Verification items for the finished model (mm, model axes). Face numbers are marked on the shaded views. A direction names the side the tool comes from. Round coordinates to 2 decimals unless told otherwise and drop trailing zeros. Write each loop counter-clockwise with the first axis right and the second up, starting at its lowest first coordinate (ties: lowest second). Pieces come first, ordered by that corner, then holes. Notation, with made-up numbers: M 76.5,14 L 118.5,14 A20 ccw 118.5,28 Z; hole C 8.25,30 d5. An arc over 180 degrees is marked long. Answer in a Markdown table with one row per item. Add a question column.
1. Set-up check for the marked faces 1, 2 and 3: record each of +Z, -Z, +X, -X, +Y, -Y from which the full face is reachable in a straight line by a thin tool's end or side.
2. Material ranges on probe 1 along Y at (x, z) = (38.5, 1.35); probe 2 along X at (y, z) = (-0.25, 16.25); probe 3 along Z at (x, y) = (-35, -3), recorded low to high.
3. Sectioned sample at D-D on z = 6.5. Record the cut outline in (x, y).
4. Sectioned sample at B-B on y = -3. Record the cut outline in (x, z).
5. Go/stop test with flat-tipped pins: pin 1 Ø2 at (x, z) = (18.5, 1.5) entering from +Y; pin 2 Ø1.5 at (y, z) = (-1, 4) entering from -X; pin 3 Ø6 at (y, z) = (6, 9) entering from -X; pin 4 Ø2 at (x, y) = (-38.5, -6.5) entering from -Z. Record where each tip stops, or that it passes through.
6. Draft check along X on the marked faces 4 and 5. Enter one of: pulls with the +X half, pulls with the -X half, needs draft (parallel to the pull), parting line crosses it, or undercut.
7. Sectioned sample at C-C on x = 26. Record the cut outline in (y, z).
8. Sectioned sample at A-A on x = -38.5. Record the cut outline in (y, z).
```python
from build123d import *

# Parameters (mm, degrees)
SKETCH_1_W            = 80
SKETCH_1_H            = 16
EXTRUDE_404_DEPTH     = 2
SKETCH_5_R            = 1.25
CUT_EXTRUDE_623_DEPTH = 41.841155713
SKETCH_3_W            = 13
SKETCH_3_H            = 13
EXTRUDE_867_DEPTH     = 3
SKETCH_4_R            = 5
EXTRUDE_1060_DEPTH    = 12
SKETCH_2_W            = 9
SKETCH_2_H            = 6
MICROUSB_DEPTH        = 3


with BuildPart() as part:
    # Эскиз1 → Extrude 404 (new body)
    with BuildSketch(Plane.XY):
        Rectangle(SKETCH_1_W, SKETCH_1_H)
    extrude(amount=EXTRUDE_404_DEPTH)

    # Эскиз5 → Cut-Extrude 623 (cut, through all)
    with BuildSketch(Plane.XY.offset(2)):
        with Locations((-38.5, 6.5)):
            Circle(SKETCH_5_R)
        with Locations((38.5, 6.5)):
            Circle(SKETCH_5_R)
        with Locations((38.5, -6.5)):
            Circle(SKETCH_5_R)
        with Locations((-38.5, -6.5)):
            Circle(SKETCH_5_R)
    extrude(amount=-CUT_EXTRUDE_623_DEPTH, mode=Mode.SUBTRACT)

    # Эскиз3 → Extrude 867 (add)
    with BuildSketch(Plane.XY.offset(2)):
        with Locations((-30, 0)):
            Rectangle(SKETCH_3_W, SKETCH_3_H)
    extrude_867 = extrude(amount=EXTRUDE_867_DEPTH)

    # Эскиз4 → Extrude 1060 (add)
    with BuildSketch(Plane.XY.offset(5)):
        with Locations(Location((-30, 0, 0), (0, 0, 180))):
            Circle(SKETCH_4_R)
    extrude_1060 = extrude(amount=EXTRUDE_1060_DEPTH)

    # Зеркальное отражение1: Extrude 867, Extrude 1060 across plane
    add(extrude_867.mirror(Plane(origin=(0, 0, 0), x_dir=(0, 0, 1), z_dir=(1, 0, 0))))
    add(extrude_1060.mirror(Plane(origin=(0, 0, 0), x_dir=(0, 0, 1), z_dir=(1, 0, 0))))

    # Эскиз2 → microusb (add)
    with BuildSketch(Plane.XY.offset(2)):
        with Locations((0, 6)):
            Rectangle(SKETCH_2_W, SKETCH_2_H)
    extrude(amount=MICROUSB_DEPTH)


solid = part.part
```
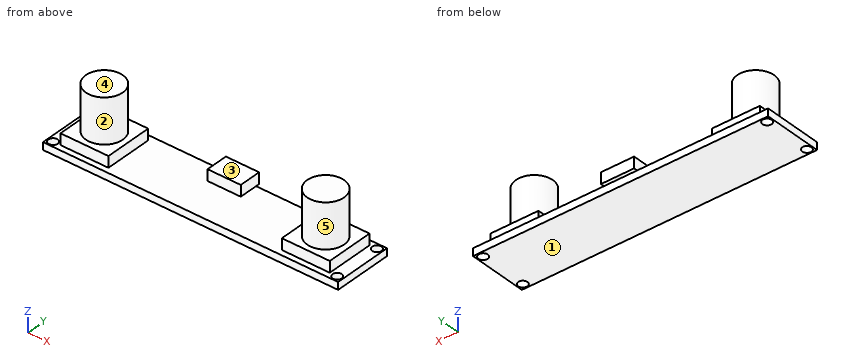
Geometry check:
| question | item | result |
|---|---|---|
| 1 | face 1 | -Z, +X, -X, +Y, -Y |
| 1 | face 2 | +Z |
| 1 | face 3 | +Z, +Y, -Y |
| 2 | probe 1 | y = -8 to -7.75, -5.25 to 5.25, 7.75 to 8 |
| 2 | probe 2 | x = -34.99 to -25.01, 25.01 to 34.99 |
| 2 | probe 3 | z = 0 to 5 |
| 3 | outline | C -30,0 d10; C 30,0 d10 |
| 4 | outline | M -40,0 L 40,0 L 40,2 L 36.5,2 L 36.5,5 L 34,5 L 34,17 L 26,17 L 26,5 L 23.5,5 L 23.5,2 L -23.5,2 L -23.5,5 L -26,5 L -26,17 L -34,17 L -34,5 L -36.5,5 L -36.5,2 L -40,2 Z |
| 5 | pin 1 | stops at y = 8 |
| 5 | pin 2 | stops at x = -36.5 |
| 5 | pin 3 | stops at x = -34 |
| 5 | pin 4 | passes through |
| 6 | face 4 | needs draft |
| 6 | face 5 | undercut |
| 7 | outline | M -8,0 L 8,0 L 8,2 L 6.5,2 L 6.5,5 L 3,5 L 3,17 L -3,17 L -3,5 L -6.5,5 L -6.5,2 L -8,2 Z |
| 8 | outline | M -8,0 L -7.75,0 L -7.75,2 L -8,2 Z; M -5.25,0 L 5.25,0 L 5.25,2 L -5.25,2 Z; M 7.75,0 L 8,0 L 8,2 L 7.75,2 Z |
